```python
from build123d import *

# Parameters (mm, degrees)
SKETCH2_R                = 20
BOSS_EXTRUDE1_DEPTH      = 14
SKETCH3_R                = 12
SKETCH3_R_2              = 6.5
EXTRUDE_THIN1_DEPTH      = 2
FILLET1_R                = 2
BOSS_EXTRUDE4_REACH      = 34.496
BOSS_EXTRUDE4_END_RADIUS = 21
SKETCH4_W                = 14
SKETCH4_H                = 1
BOSS_EXTRUDE5_DEPTH      = 23
SKETCH6_W                = 6
SKETCH6_H                = 7
BOSS_EXTRUDE6_DEPTH      = 21
BOSS_EXTRUDE7_DEPTH      = 20
BOSS_EXTRUDE8_START      = 16
SKETCH8_R                = 11
BOSS_EXTRUDE8_DEPTH      = 6
SHELL1_START             = 10
SHELL1_DEPTH             = 2
SHELL1_START_2           = -1.5
SHELL1_2_DEPTH           = 23.5
SHELL1_START_3           = 18
SHELL1_3_DEPTH           = 4
SHELL1_START_4           = 2
SHELL1_4_DEPTH           = 10
CUT_EXTRUDE1_REACH       = 38.565
BOSS_EXTRUDE9_DEPTH      = 7
BOSS_EXTRUDE10_DEPTH     = 28
FILLET2_R                = 1


with BuildPart() as part:
    # Sketch2 → Boss-Extrude1 (new body)
    with BuildSketch(Plane(origin=(0, 0, 0), x_dir=(0, 0, -1), z_dir=(1, 0, 0))):
        Circle(SKETCH2_R)
    extrude(amount=BOSS_EXTRUDE1_DEPTH)

    # Sketch3 → Extrude-Thin1 (add)
    with BuildSketch(Plane(origin=(14, 0, 0), x_dir=(0, 0, -1), z_dir=(1, 0, 0))):
        Circle(SKETCH3_R)
        Circle(SKETCH3_R_2, mode=Mode.SUBTRACT)
    extrude(amount=EXTRUDE_THIN1_DEPTH)

    # Fillet1
    fillet1_edges = [part.edges().sort_by_distance(p)[0] for p in [
        (16, 0, 12),
        (16, 0, 6.5),
    ]]
    fillet(fillet1_edges, radius=FILLET1_R - 0.0001)  # a hair under: the kernel refuses the full size

    # Boss-Extrude4: up to this cylinder (the profile starts inside it)
    boss_extrude4_end = Plane(origin=(7, 0, 0), z_dir=(-1, 0, 0)) * Cylinder(BOSS_EXTRUDE4_END_RADIUS, 111.992, mode=Mode.PRIVATE)
    # Sketch4 → Boss-Extrude4 (add, up to the surface)
    with BuildSketch(Plane(origin=(0, 0, 0), x_dir=(1, 0, 0), z_dir=(0, 1, 0)), mode=Mode.PRIVATE) as boss_extrude4_sk1:
        with Locations((7, 7)):
            Rectangle(SKETCH4_W, SKETCH4_H)
    boss_extrude4_tool1 = extrude(boss_extrude4_sk1.sketch, amount=BOSS_EXTRUDE4_REACH, mode=Mode.PRIVATE) & boss_extrude4_end
    add(boss_extrude4_tool1.solids().sort_by_distance((7, 0, -7))[0])
    # Sketch4 → Boss-Extrude4 (add, up to the surface)
    with BuildSketch(Plane(origin=(0, 0, 0), x_dir=(1, 0, 0), z_dir=(0, 1, 0)), mode=Mode.PRIVATE) as boss_extrude4_sk2:
        with Locations((7, -7)):
            Rectangle(SKETCH4_W, SKETCH4_H)
    boss_extrude4_tool2 = extrude(boss_extrude4_sk2.sketch, amount=BOSS_EXTRUDE4_REACH, mode=Mode.PRIVATE) & boss_extrude4_end
    add(boss_extrude4_tool2.solids().sort_by_distance((7, 0, 7))[0])

    # Sketch5 → Boss-Extrude5 (add)
    with BuildSketch(Plane(origin=(0, 0, 0), x_dir=(1, 0, 0), z_dir=(0, 1, 0))):
        Polygon((2, 6.5), (2, -6.5), (14, -6.5), (14, -7.5), (0, -7.5), (0, 7.5), (14, 7.5), (14, 6.5), align=None)
    extrude(amount=-BOSS_EXTRUDE5_DEPTH)

    # Sketch6 → Boss-Extrude6 (add)
    with BuildSketch(Plane(origin=(0, 0, 0), x_dir=(1, 0, 0), z_dir=(0, 1, 0))):
        with Locations((11, 0)):
            Rectangle(SKETCH6_W, SKETCH6_H)
    extrude(amount=-BOSS_EXTRUDE6_DEPTH)

    # Sketch7 → Boss-Extrude7 (add)
    with BuildSketch(Plane.XY):
        Polygon((0, 7.5), (14, 7.5), (14, 6.5), (2, 6.5), (2, -6.5), (14, -6.5), (14, -7.5), (0, -7.5), align=None)
    extrude(amount=-BOSS_EXTRUDE7_DEPTH)

    # Sketch8 → Boss-Extrude8 (add)
    with BuildSketch(Plane.XY.offset(BOSS_EXTRUDE8_START)):
        with Locations(Location((7, 0, 0), (0, 0, 129.521196359))):
            Circle(SKETCH8_R)
    extrude(amount=BOSS_EXTRUDE8_DEPTH)

    # Shell1: read off the stored shape, not the designer's step
    # Shell1 outline → Shell1 (cut)
    with BuildSketch(Plane.YZ.offset(SHELL1_START)):
        with BuildLine():
            Line((-19, -1.5), (-17.937391115, -1.5))
            ThreePointArc((-17.937391115, -1.5), (-18, 0), (-17.937391115, 1.5))
            Line((-17.937391115, 1.5), (-19, 1.5))
            Line((-19, 1.5), (-19, -1.5))
        make_face()
    extrude(amount=SHELL1_DEPTH, mode=Mode.SUBTRACT)

    # Shell1 2 outline → Shell1 2 (cut)
    with BuildSketch(Plane.XY.offset(SHELL1_START_2)):
        with BuildLine():
            Line((2, 7.483314774), (2, -7.483314774))
            ThreePointArc((2, -7.483314774), (7, -9), (12, -7.483314774))
            Line((12, -7.483314774), (12, 7.483314774))
            ThreePointArc((12, 7.483314774), (7, 9), (2, 7.483314774))
        make_face()
    extrude(amount=SHELL1_2_DEPTH, mode=Mode.SUBTRACT)

    # Shell1 3 outline → Shell1 3 (cut)
    with BuildSketch(Plane.XY.offset(SHELL1_START_3)):
        with BuildLine():
            ThreePointArc((2, 7.483314774), (-2, 0), (2, -7.483314774))
            Line((2, -7.483314774), (2, 7.483314774))
        make_face()
        with BuildLine():
            Line((12, 7.483314774), (12, -7.483314774))
            ThreePointArc((12, -7.483314774), (16, 0), (12, 7.483314774))
        make_face()
    extrude(amount=SHELL1_3_DEPTH, mode=Mode.SUBTRACT)

    # Shell1 4 outline → Shell1 4 (cut)
    with BuildSketch(Plane.YZ.offset(SHELL1_START_4)):
        with BuildLine():
            Line((7.483314774, 16.370705544), (3.91902534, 18))
            Line((3.91902534, 18), (-3.91902534, 18))
            Line((-3.91902534, 18), (-7.483314774, 16.370705544))
            ThreePointArc((-7.483314774, 16.370705544), (0, -18), (7.483314774, 16.370705544))
        make_face()
    extrude(amount=SHELL1_4_DEPTH, mode=Mode.SUBTRACT)

    # Sketch9 → Cut-Extrude1 (cut, up to next)
    with BuildSketch(Plane(origin=(14, 0, 0), x_dir=(0, 0, -1), z_dir=(1, 0, 0)), mode=Mode.PRIVATE) as cut_extrude1_sk1:
        with BuildLine():
            ThreePointArc((0, 6.5), (-4.596194078, 4.596194078), (-6.5, 0))
            ThreePointArc((-6.5, 0), (-4.596194078, -4.596194078), (0, -6.5))
            ThreePointArc((0, -6.5), (4.596194078, -4.596194078), (6.5, 0))
            ThreePointArc((6.5, 0), (4.596194078, 4.596194078), (0, 6.5))
        make_face()
    cut_extrude1_tool1 = extrude(cut_extrude1_sk1.sketch, amount=-CUT_EXTRUDE1_REACH, mode=Mode.PRIVATE) & part.part
    add(cut_extrude1_tool1.solids().sort_by_distance((14, 0, 0))[0], mode=Mode.SUBTRACT)

    # Sketch10 → Boss-Extrude9 (add)
    with BuildSketch(Plane.ZY):
        with BuildLine():
            Line((7, 9), (-7, 9))
            ThreePointArc((-7, 9), (-11, 0), (-7, -9))
            Line((-7, -9), (7, -9))
            ThreePointArc((7, -9), (11, 0), (7, 9))
        make_face()
    extrude(amount=BOSS_EXTRUDE9_DEPTH)

    # Sketch11 → Boss-Extrude10 (add)
    with BuildSketch(Plane.ZY.offset(7)):
        with BuildLine():
            Line((-6.5, -7.5), (6.5, -7.5))
            ThreePointArc((6.5, -7.5), (10, 0), (6.5, 7.5))
            Line((6.5, 7.5), (-6.5, 7.5))
            ThreePointArc((-6.5, 7.5), (-10, 0), (-6.5, -7.5))
        make_face()
    extrude(amount=BOSS_EXTRUDE10_DEPTH)

    # Fillet2
    fillet2_edges = [part.edges().sort_by_distance(p)[0] for p in [
        (-21, -7.5, 6.5),
        (-21, 7.5, 6.5),
        (-21, 7.5, -6.5),
        (-21, -7.5, -6.5),
    ]]
    fillet(fillet2_edges, radius=FILLET2_R)


solid = part.part
```
Can you work these out from the model? Positions are in its coordinate system, mm. A direction names the side the tool comes from. Give positions to 0.01 mm unless a question says otherwise; leave off trailing zeros. Write each loop counter-clockwise with the first axis right and the second up, starting at its lowest first coordinate (ties: lowest second). Pieces come first, ordered by that corner, then holes. Notation, with made-up numbers: (39, 18) -> (77, 18) arc R13 ccw to (77, 39) -> close; hole circle Ø7 at (84, 45). An arc over 180 degrees is marked (long way). Write item = value, one per line.
(1) I'm going to push flat-ended pins straight in: P1, Ø0.5, axis at x = 5.5, z = -19.5, coming from the -Y side; P2, Ø2, axis at x = -2, z = -2.5, coming from the +Y side; P3, Ø8, axis at x = -17, y = -15, coming from the -Z side; P4, Ø0.8, axis at x = 5.5, y = 19.5, coming from the -Z side. Where does each tip first touch, or does it pass through?
Worked out:
P1 = -7.5
P2 = 9
P3 = through
P4 = -7.5
(2) I need wall thicknesses on probe 1 along Y at (x, z) = (6, 0); probe 2 along X at (y, z) = (-2, -10); probe 3 along X at (y, z) = (4, -16). Which ranges of each line are inside material? Lowest first, please. Write a range as from..to.
Worked out:
probe_1 = -20..-18, 18..20
probe_2 = -7..2, 12..15.99
probe_3 = 0..2, 12..14
(3) Suppose I cut it at B-B on y = -14. Write out the boundary of the cut face in (x, z).
Worked out:
outline = (0, -14.28) -> (14, -14.28) -> (14, 14.28) -> (0, 14.28) -> close; hole (2, -11.31) -> (12, -11.31) -> (12, 11.31) -> (2, 11.31) -> close
(4) Suppose I cut it at D-D on z = -13. Write out the boundary of the cut face in (x, y), then the cut area to 3 significant figures.
Worked out:
outline = (0, -15.2) -> (14, -15.2) -> (14, 15.2) -> (0, 15.2) -> close; hole (2, -12.45) -> (12, -12.45) -> (12, 12.45) -> (2, 12.45) -> close
area = 177 mm^2
(5) Suppose I cut it at C-C on x = -12. Write out the boundary of the cut face in (y, z).
Worked out:
outline = (-7.5, -6.13) arc R1 ccw to (-7.24, -6.8) arc R9.79 ccw to (7.24, -6.8) arc R1 ccw to (7.5, -6.13) -> (7.5, 6.13) arc R1 ccw to (7.24, 6.8) arc R9.79 ccw to (-7.24, 6.8) arc R1 ccw to (-7.5, 6.13) -> close
(6) Suppose I cut it at A-A on x = -1. Write out the boundary of the cut face in (y, z) (3 decimals).
Worked out:
outline = (-9, -7) arc R12.125 ccw to (9, -7) -> (9, 7) arc R12.125 ccw to (-9, 7) -> close; (-7.55, 16) -> (7.55, 16) -> (7.55, 22) -> (4.123, 22) -> (4.123, 18) -> (-4.123, 18) -> (-4.123, 22) -> (-7.55, 22) -> close
(7) For faces 4 (the face through (-21, -7.5, 0)), 5 (the face through (8, -21, 6.5)), 6 (the face through (2, -21, 0)), which set-ups out of +Z, -Z, +X, -X, +Y, -Y let a thin tool reach every point of the face, with its end or its side?
Worked out:
face_4 = +Z, -Z, -X, -Y
face_5 = +X, -Y
face_6 = -Y
(8) Thinking about a two-plate mould opening in Y: for faces 1 (the face through (0, 0, 18)), 2 (the face through (7, 7.5, -19)), 3 (the face through (16, 0, 16)), which applies, released by +Y, released by -Y, zero draft, split by the parting line, or undercut?
Worked out:
face_1 = undercut
face_2 = released by +Y
face_3 = zero draft
